Here's how the part is built. I have some questions about the finished solid (model axes, mm). A direction names the side the tool comes from. Round coordinates to 2 decimals unless told otherwise and drop trailing zeros. Order: outer loops, then holes, each group sorted by start corner. A loop starts at its lowest first (then second) coordinate and runs counter-clockwise, first axis right, second up. Notation, with made-up numbers: (88.25, -13.75) -> (122.25, -13.75) arc R9 cw to (122.25, 0.25) -> close; hole circle Ø10 at (40.25, 18.25). An arc over 180 degrees is marked (long way). Use a Markdown table: item, result. Add a question column.
(1) I want a section at B-B, the plane x = 7.5. Please give me the cut outline in (y, z), then the cut area to 3 significant figures.
(2) If I drill on probe 1 along Z at (x, y) = (0, -1.8); probe 2 along Z at (x, y) = (-1.5, -9.5), over which ranges is the centre line in solid material (lowest first)?
(3) I want a section at A-A, the plane z = 59. Please give me the cut outline in (x, y), then the cut area to 3 significant figures.
(4) Thinking about a two-plate mould opening in Z: for faces 3 (the face through (29, -4, -28.2)), 4 (the face through (-1, 0, 15)), which applies, pulls with the +Z half, pulls with the -Z half, needs draft (parallel to the pull), parting line crosses it, or undercut?
(5) I'm going to push flat-ended pins straight in: P1, Ø1.6, axis at x = 0, z = -12.5, coming from the +Y side; P2, Ø4, axis at y = -3, z = -25, coming from the -X side; P3, Ø3, axis at y = -4, z = -41, coming from the +X side; P4, Ø5.5, axis at x = -28.5, y = -4.5, coming from the +Z side. Where does each tip first touch, or does it pass through?
(6) I want a section at C-C, the plane x = 37.5. Please give me the cut outline in (y, z).
(7) On a 3-axis mill with a long thin cutter (end or side, diameter ignored), from which of +Z, -Z, +X, -X, +Y, -Y can I reach the whole of each face in a straight line? I mean faces 1 (the face through (-26.738, -4, 24)), 2 (the face through (0, -3, 5)). Say none if no direction works.
from build123d import *

# Parameters (mm, degrees)
SKETCH1_R            = 22.5
SKETCH1_R_2          = 4
SKETCH1_R_3          = 1
BOSS_EXTRUDE7_DEPTH  = 3
SKETCH1_15_R         = 67.5
SKETCH1_15_R_2       = 22.5
SKETCH1_15_W         = 5.138307475
SKETCH1_15_H         = 8
BOSS_EXTRUDE8_DEPTH  = 8
SKETCH1_20_R         = 70
SKETCH1_20_R_2       = 67.5
BOSS_EXTRUDE10_DEPTH = 11


with BuildPart() as part:
    # Sketch1 → Boss-Extrude7 (new body)
    with BuildSketch(Plane(origin=(0, 0, 0), x_dir=(1, 0, 0), z_dir=(0, 1, 0))):
        Circle(SKETCH1_R)
        Circle(SKETCH1_R_2, mode=Mode.SUBTRACT)
        with Locations((0, -12.5)):
            Circle(SKETCH1_R_3, mode=Mode.SUBTRACT)
        with Locations((0, 12.5)):
            Circle(SKETCH1_R_3, mode=Mode.SUBTRACT)
        with Locations((12.5, 0)):
            Circle(SKETCH1_R_3, mode=Mode.SUBTRACT)
        with Locations((-12.5, 0)):
            Circle(SKETCH1_R_3, mode=Mode.SUBTRACT)
    extrude(amount=-BOSS_EXTRUDE7_DEPTH)

    # Sketch1_15 → Boss-Extrude8 (add)
    with BuildSketch(Plane(origin=(0, 0, 0), x_dir=(1, 0, 0), z_dir=(0, 1, 0))):
        Circle(SKETCH1_15_R)
        Circle(SKETCH1_15_R_2, mode=Mode.SUBTRACT)
        with Locations((29.307217935, 24.2)):
            Rectangle(SKETCH1_15_W, SKETCH1_15_H, mode=Mode.SUBTRACT)
        with Locations((-29.307217935, -24.2)):
            Rectangle(SKETCH1_15_W, SKETCH1_15_H, mode=Mode.SUBTRACT)
        with Locations((-29.307217935, 24.2)):
            Rectangle(SKETCH1_15_W, SKETCH1_15_H, mode=Mode.SUBTRACT)
        with Locations((29.307217935, -24.2)):
            Rectangle(SKETCH1_15_W, SKETCH1_15_H, mode=Mode.SUBTRACT)
    extrude(amount=-BOSS_EXTRUDE8_DEPTH)

    # Sketch1_20 → Boss-Extrude10 (add)
    with BuildSketch(Plane(origin=(0, 0, 0), x_dir=(1, 0, 0), z_dir=(0, 1, 0))):
        Circle(SKETCH1_20_R)
        Circle(SKETCH1_20_R_2, mode=Mode.SUBTRACT)
    extrude(amount=-BOSS_EXTRUDE10_DEPTH)


solid = part.part
Taken from the geometry:
| question | item | result |
|---|---|---|
| 1 | outline | (-11, -69.6) -> (0, -69.6) -> (0, 69.6) -> (-11, 69.6) -> (-11, 67.08) -> (-8, 67.08) -> (-8, 21.21) -> (-3, 21.21) -> (-3, -21.21) -> (-8, -21.21) -> (-8, -67.08) -> (-11, -67.08) -> close |
| 1 | area | 917 mm2 |
| 2 | probe 1 | z = -70 to -13.5, -11.5 to -4, 4 to 11.5, 13.5 to 70 |
| 2 | probe 2 | z = -69.98 to -67.48, 67.48 to 69.98 |
| 3 | outline | (-37.67, -11) -> (-32.79, -11) -> (-32.79, -8) -> (32.79, -8) -> (32.79, -11) -> (37.67, -11) -> (37.67, 0) -> (-37.67, 0) -> close |
| 3 | area | 632 mm2 |
| 4 | face 3 | undercut |
| 4 | face 4 | needs draft |
| 5 | P1 | passes through |
| 5 | P2 | stops at x = -66.11 |
| 5 | P3 | stops at x = 57.79 |
| 5 | P4 | stops at z = 65.09 |
| 6 | outline | (-11, -59.11) -> (0, -59.11) -> (0, 59.11) -> (-11, 59.11) -> (-11, 56.12) -> (-8, 56.12) -> (-8, -56.12) -> (-11, -56.12) -> close |
| 7 | face 1 | +Y, -Y |
| 7 | face 2 | -Y |
